Source: CAD feature listing. Evaluate the final solid. Frame: model axes, mm. Face numbers are marked on the shaded views. A direction names the side the tool comes from. Round coordinates to 2 decimals unless told otherwise and drop trailing zeros. Loops run counter-clockwise (first coordinate to the right, second up) from the corner with the lowest first, then second, coordinate; pieces in that order, holes last. Notation, with made-up numbers: (-7, -18) - (-3, -18) arc R16 ccw to (-3, 13) - close; hole circle Ø6 at (-28.75, 29). An arc over 180 degrees is marked (long way). Use CSV: the item, a comma, the result in double quotes. Start each with the question number.
from build123d import *

# Parameters (mm, degrees)
SKETCH1_W           = 80
SKETCH1_H           = 20
SKETCH1_R           = 2.5
BOSS_EXTRUDE1_DEPTH = 2
SKETCH2_R           = 2
BOSS_EXTRUDE2_DEPTH = 23


with BuildPart() as part:
    # Sketch1 → Boss-Extrude1 (new body)
    with BuildSketch(Plane.XY):
        with Locations((-9.925787146, -16.395190745)):
            Rectangle(SKETCH1_W, SKETCH1_H)
        with Locations((-37.425787146, -16.395190745)):
            Circle(SKETCH1_R, mode=Mode.SUBTRACT)
        with Locations((17.574212854, -16.395190745)):
            Circle(SKETCH1_R, mode=Mode.SUBTRACT)
    extrude(amount=BOSS_EXTRUDE1_DEPTH)

    # Sketch2 → Boss-Extrude2 (add)
    with BuildSketch(Plane.XY.offset(2)):
        with Locations((25.074212854, -16.395190745)):
            Circle(SKETCH2_R)
        with Locations((-44.925787146, -16.395190745)):
            Circle(SKETCH2_R)
    extrude(amount=BOSS_EXTRUDE2_DEPTH)


solid = part.part
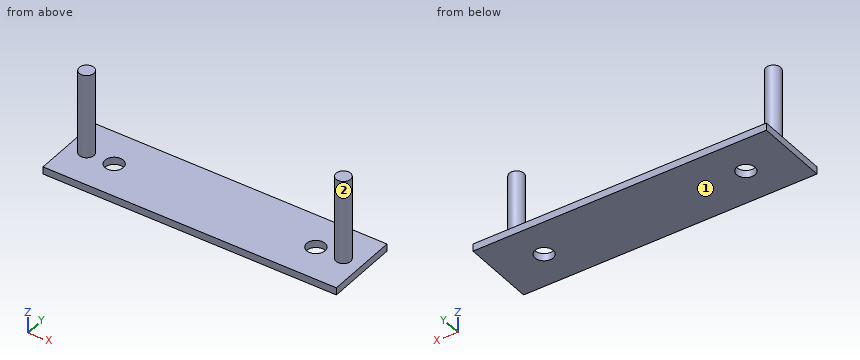
1. Reachability of the marked faces 1 and 2 from +Z, -Z, +X, -X, +Y, -Y: full face, straight path, thin tool, end or side. Return the list, or none.
2. Section query C-C on x = 6. Return the cut outline in (y, z).
3. Contact query for flat-ended pins moving along their axis: P1, Ø2, axis at x = 13, y = -11, coming from the +Z side; P2, Ø4, axis at x = -20, y = -19, coming from the -Z side; P3, Ø10, axis at x = -39, z = 21.5, coming from the -Y side. Output: stop coordinate, or through.
4. Section query B-B on y = -23.5. Return the cut outline in (x, z).
5. Section query D-D on z = 23.5. Return the cut outline in (x, y).
6. Section query A-A on y = -15.5. Return the cut outline in (x, z), and give its area (3 significant figures).
7. Line query: line 1 along Z through (x, y) = (11, -22.5); line 2 along X through (y, z) = (-17.75, 11.5). Output: solid intervals per line, ascending.
Values:
1,face 1,"-Z, +X, -X, +Y, -Y"
1,face 2,"+Z"
2,outline,"(-26.4, 0) - (-6.4, 0) - (-6.4, 2) - (-26.4, 2) - close"
3,P1,"stops at z = 2"
3,P2,"stops at z = 0"
3,P3,"stops at y = -18.17"
4,outline,"(-49.93, 0) - (30.07, 0) - (30.07, 2) - (-49.93, 2) - close"
5,outline,"circle Ø4 at (-44.93, -16.4); circle Ø4 at (25.07, -16.4)"
6,outline,"(-49.93, 0) - (-39.76, 0) - (-39.76, 2) - (-43.14, 2) - (-43.14, 25) - (-46.71, 25) - (-46.71, 2) - (-49.93, 2) - close; (-35.09, 0) - (15.24, 0) - (15.24, 2) - (-35.09, 2) - close; (19.91, 0) - (30.07, 0) - (30.07, 2) - (26.86, 2) - (26.86, 25) - (23.29, 25) - (23.29, 2) - (19.91, 2) - close"
6,area,"306 mm^2"
7,line 1,"z = 0 to 2"
7,line 2,"x = -46.4 to -43.45, 23.6 to 26.55"
